Autodesk Inventor part; units mm, degrees
ref_plane "YZ Plane" through (0, 0, 0) normal (1, 0, 0) x (0, 1, 0)
ref_plane "XZ Plane" through (0, 0, 0) normal (0, 1, 0) x (-1, 0, 0)
ref_plane "XY Plane" through (0, 0, 0) normal (0, 0, 1) x (1, 0, 0)
ref_plane "Plano de trabajo1" through (0, 0, 0) normal (0, 0, 1) x (1, 0, 0)
sketch "Boceto1" plane through (0, 0, 0) normal (0, 0, 1) x (1, 0, 0)
  circle A0 centre (10.9923, 0) radius 10.9823
  circle A1 centre (10.9923, 0) radius 3.1378
  circle A2 centre (18.3423, 0) radius 1.2028
  circle A3 centre (10.9923, 7.35) radius 1.2028
  circle A4 centre (3.6423, 0) radius 1.2028
  circle A5 centre (10.9923, -7.35) radius 1.2028
  line L0 (0, 0) -> (0, 30)
  line L1 (21.9746, 0) -> (21.9746, -30)
  line L2 (0, 0) -> (0, -30)
  line L3 (0, -30) -> (21.9746, -30)
  circle A6 centre (10.9923, 0) radius 3.1378
  circle A7 centre (18.3423, 0) radius 1.2028
  circle A8 centre (10.9923, -7.35) radius 1.2028
  circle A9 centre (3.6423, 0) radius 1.2028
  circle A10 centre (10.9923, 7.35) radius 1.2028
  circle A11 centre (10.9923, 0) radius 10.9823
  line L4 (0, 0) -> (0, -30)
  line L5 (0, -30) -> (21.9746, -30)
  line L6 (21.9746, -30) -> (21.9746, 0)
  dimension "d0" = 30
  dimension "d1" = 30
extrude "Extrusión1" add sketch "Boceto1" along normal blind 3
sketch "Boceto2" plane through (10.9923, 0, 3) normal (0, 0, 1) x (1, 0, 0)
  circle A0 centre (0, 0) radius 10.9823
  line L0 (10.9823, 0) -> (10.9823, -30)
  line L1 (10.9823, -30) -> (-9.7118, -30)
  line L2 (-9.7118, -30) -> (-10.9923, 0)
  circle A1 centre (0, 0) radius 10.9823
  circle A2 centre (0, -7.35) radius 1.2028
  circle A3 centre (-7.35, 0) radius 1.2028
  circle A4 centre (0, 7.35) radius 1.2028
  circle A5 centre (7.35, 0) radius 1.2028
  circle A6 centre (0, 0) radius 3.1378
  point P0 (-10.9723, -0.4683)
  dimension "d4" = 30
extrude "Extrusión2" add sketch "Boceto2" against normal blind 3 contours L0 L1 L2 A0
sketch "Boceto3" plane through (0, 0, 0) normal (0, 0, -1) x (-1, 0, 0)
  point P0 (0, 0)
sketch "Boceto4" plane through (0, 0, 3) normal (0, 0, 1) x (1, 0, 0)
  point P0 (0, 0)
sketch "Boceto5" plane through (0, 0, 0) normal (0, 0, -1) x (-1, 0, 0)
  arc A0 (-0.02, -0.4683) -> (-21.9746, 0) centre (-10.9923, 0) ccw
  line L0 (-21.9746, 0) -> (-21.9746, -30)
  line L1 (-21.9746, -30) -> (-1.2805, -30)
  line L2 (-1.2805, -30) -> (-0.02, -0.4683)
  circle A1 centre (-10.9923, -7.35) radius 1.2028
  circle A2 centre (-3.6423, 0) radius 1.2028
  circle A3 centre (-10.9923, 7.35) radius 1.2028
  circle A4 centre (-18.3423, 0) radius 1.2028
  circle A5 centre (-10.9923, 0) radius 3.1378
  line L3 (-21.9746, -30) -> (0, -30)
  line L4 (0, -30) -> (0, 0)
  line L5 (0, 0) -> (-21.9746, 0)
  line L6 (-21.9746, 0) -> (-21.9746, -30)
  point P0 (-0.01, 0)
extrude "Extrusión3" add sketch "Boceto5" against normal blind 3 contours A0 L5 L4 L3 L2
sketch "Boceto6" plane through (0, 0, 0) normal (0, 0, -1) x (-1, 0, 0)
  point P0 (0, 0)
sketch "Boceto7" plane through (0, 0, 0) normal (0, 0, -1) x (-1, 0, 0)
  line L0 (-21.9746, -30) -> (0, -30)
  line L1 (-21.9746, -30) -> (-21.9746, 0)
  line L2 (0, -30) -> (-21.9746, -30)
  line L3 (-21.9746, -30) -> (-21.9746, -27)
  line L4 (-21.9746, -27) -> (0, -27)
  line L5 (0, -27) -> (0, -30)
  point P0 (0, 0)
  dimension "d9" = 3
extrude "Extrusión4" add sketch "Boceto7" along normal blind 40
sketch "Boceto8" plane through (0, -27, 0) normal (0, 1, 0) x (1, 0, 0)
  line L0 (0, -3) -> (0, 40)
  line L1 (21.9746, -3) -> (21.9746, 40)
  line L2 (0, 40) -> (21.9746, 40)
  line L3 (21.9746, 40) -> (21.9746, 38)
  line L4 (21.9746, 38) -> (0, 38)
  line L5 (0, 38) -> (0, 40)
  point P0 (0, 0)
  point P1 (21.9746, 40)
  point P2 (0, 38)
  dimension "d12" = 2
extrude "Extrusión5" add sketch "Boceto8" along normal blind 40
sketch "Boceto9" plane through (0, 0, -40) normal (0, 0, -1) x (-1, 0, 0)
  circle A0 centre (-11.0072, -0.015) radius 2.7
  circle A1 centre (-11.0099, -0.0117) radius 10.9823
  circle A2 centre (-18.3423, 0) radius 1.2028
  circle A3 centre (-10.9923, -7.35) radius 1.2028
  circle A4 centre (-10.9923, 7.35) radius 1.2028
  circle A5 centre (-3.6423, 0) radius 1.2028
  line L0 (-21.9746, -30) -> (-21.9746, 13)
  line L1 (-21.9746, -30) -> (0, -30)
  line L2 (0, -30) -> (0, 13)
  line L3 (-21.9746, 13) -> (0, 13)
  line L4 (-21.5706, 0) -> (-25.972, 0)
  line L5 (-25.972, 0) -> (-25.972, 18.1609)
  line L6 (-25.972, 18.1609) -> (4.5124, 18.1609)
  line L7 (4.5124, 18.1609) -> (4.5124, 1.2028)
  line L8 (4.5124, 1.2028) -> (4.5124, 0)
  line L9 (-3.6423, 0) -> (4.822, 0)
  point P0 (0, 0)
  point P1 (-21.9746, 0.6093)
  point P2 (-0.0276, 0)
  point P3 (0, 0)
extrude "Extrusión6" cut sketch "Boceto9" against normal blind 40 contours A0 | A1 L0 L3 L2 L9 | A2 | A3 | A4 | A5
sketch "Boceto10" plane through (0, -30, 3) normal (0, -1, 0) x (1, 0, 0)
  point P0 (0, -3)
sketch "Boceto11" plane through (0, -30, 3) normal (0, -1, 0) x (1, 0, 0)
  line L0 (0.0276, -43) -> (21.9746, -43)
  line L1 (0, -3) -> (0, 0)
  line L2 (21.9746, -43) -> (0, -43)
  line L3 (0, -43) -> (0, 0)
  line L4 (0, 0) -> (21.9746, 0)
  line L5 (21.9746, 0) -> (21.9746, -43)
  line L6 (0, -43) -> (-100, -43)
  line L7 (-100, -43) -> (-100, 0)
  line L8 (-100, 0) -> (0, 0)
  line L9 (0, 0) -> (0, -43)
  line L10 (-100, 0) -> (-100, -21.5)
  line L11 (-100, -21.5) -> (-100, -14.5)
  line L12 (-100, -14.5) -> (-100, -28.5)
  line L13 (-100, -28.5) -> (-50, -43)
  line L14 (-50, -43) -> (-50, 0)
  line L15 (-100, -14.5) -> (-50, 0)
  dimension "d17" = 100
  dimension "d18" = 21.5
  dimension "d19" = 7
  dimension "d20" = 14
extrude "Extrusión7" add sketch "Boceto11" along normal blind 10 contours L2 L3 L1 L4 L5 L0 | L6 L14 L8 L1 L3 | L13 L7 L15 L14
chamfer "Chaflán1" distance 2 angle 45 12 edges at (-14.0127, -40, -40) (-75, -40, -32.75) (-75, -30, -32.75) (-25, -30, -40) (-14.0127, -40, 3) (-75, -40, -4.25) (-100, -40, -18.5) (-75, -30, -4.25) (-25, -30, 3) (-100, -30, -18.5) (-100, -35, -25.5) (-100, -35, -11.5)
sketch "Boceto12" plane through (0, -40, 3) normal (0, -1, 0) x (1, 0, 0)
  line L0 (-49.7159, -2) -> (21.9746, -2)
  line L1 (-98, -16.0024) -> (-49.7159, -2)
  line L2 (-98, -26.9976) -> (-98, -16.0024)
  line L3 (-49.7159, -41) -> (-98, -26.9976)
  line L4 (21.9746, -41) -> (-49.7159, -41)
  line L5 (21.9746, -41) -> (21.9746, -2)
  line L6 (-48.5793, -33) -> (-88.2344, -21.5)
  line L7 (-88.2344, -21.5) -> (-48.5793, -10)
  line L8 (-48.5793, -10) -> (13.9746, -10)
  line L9 (13.9746, -10) -> (13.9746, -33)
  line L10 (13.9746, -33) -> (-48.5793, -33)
  point P0 (0, -3)
  dimension "d26" = 8
extrude "Extrusión8" cut sketch "Boceto12" against normal blind 4 contours L6 L7 L8 L9 L10
sketch "Boceto13" plane through (0, 0, -40) normal (0, 0, -1) x (-1, 0, 0)
  circle A0 centre (-11.0099, -0.0117) radius 5.6
  circle A1 centre (-11.0072, -0.015) radius 2.7
  point P0 (0, 0)
extrude "Extrusión9" cut sketch "Boceto13" against normal blind 5
sketch "Boceto14" plane through (0, 0, 0) normal (-1, 0, 0) x (0, 0, 1)
  line L0 (0, -27) -> (-38, -27)
  line L1 (-38, 0) -> (-40, 0)
  line L2 (-40, -32) -> (-40, 0)
  line L3 (-38, -30) -> (-40, -32)
  line L4 (1, -30) -> (-38, -30)
  line L5 (3, -32) -> (1, -30)
  line L6 (3, 0) -> (3, -32)
  line L7 (0, 0) -> (3, 0)
  line L8 (0, -27) -> (0, 0)
  line L9 (0, -27) -> (-38, -27)
  line L10 (-38, -27) -> (-38, 0)
  point P0 (0, 0)
extrude "Extrusión10" add sketch "Boceto14" along normal blind 30
sketch "Boceto15" plane through (0, 0, 3) normal (0, 0, 1) x (1, 0, 0)
  line L0 (21.9746, -38) -> (-50, -38)
  line L1 (21.9746, -38) -> (21.9746, 0)
  arc A0 (21.9746, 0) -> (0.01, 0) centre (10.9923, 0) ccw
  line L2 (0.01, 0) -> (-30, 0)
  line L3 (-30, -32) -> (-30, 0)
  line L4 (-50, -32) -> (-30, -32)
  line L5 (-50, -32) -> (-50, -38)
  circle A1 centre (10.9923, -7.35) radius 1.2028
  circle A2 centre (3.6423, 0) radius 1.2028
  circle A3 centre (10.9923, 7.35) radius 1.2028
  circle A4 centre (18.3423, 0) radius 1.2028
  circle A5 centre (10.9923, 0) radius 3.1378
  line L6 (21.9746, -27) -> (-30, -27)
  line L7 (0.01, 0) -> (-30, -27)
  point P0 (0, 0)
extrude "Extrusión11" cut sketch "Boceto15" against normal blind 100 contours L3 L2 L7
chamfer "Chaflán2" distance 2 angle 45 1 edges at (-30, -27, -19)
sketch "Boceto16" plane through (21.9746, -27, 0) normal (0, 1, 0) x (1, 0, 0)
  line L0 (-49.9746, 0) -> (-49.9746, 38)
  line L1 (0, 0) -> (-49.9746, 0)
  line L2 (0, 0) -> (0, 38)
  line L3 (0, 38) -> (-49.9746, 38)
  line L4 (0, 0) -> (-16, 0)
  line L5 (-16, 0) -> (-16, 6)
  line L6 (-16, 6) -> (0, 6)
  line L7 (0, 6) -> (0, 0)
  line L8 (0, 38) -> (-16, 38)
  line L9 (-16, 38) -> (-16, 32)
  line L10 (-16, 32) -> (0, 32)
  line L11 (0, 32) -> (0, 38)
  point P0 (-21.9746, 0)
  dimension "d38" = 16
  dimension "d39" = 6
  dimension "d40" = 16
  dimension "d41" = 6
extrude "Extrusión12" add sketch "Boceto16" along normal blind 6 contours L5 L6 L2 L1 | L3 L2 L10 L9
chamfer "Chaflán3" distance 6 angle 45 2 edges at (13.9746, -21, -6) (13.9746, -21, -32)
sketch "Boceto17" plane through (5.9746, -27, -38) normal (-1, 0, 0) x (0, 0, 1)
  line L0 (0, 6) -> (6, 0)
  line L1 (0, 0) -> (0, 6)
  line L2 (6, 0) -> (0, 0)
  line L3 (32, 0) -> (38, 6)
  line L4 (38, 0) -> (32, 0)
  line L5 (38, 6) -> (38, 0)
  point P0 (38, 27)
extrude "Extrusión13" add sketch "Boceto17" along normal blind 28
sketch "Boceto18" plane through (0, 0, -40) normal (0, 0, -1) x (-1, 0, 0)
  circle A0 centre (-10.9923, 0) radius 3.1378
  circle A1 centre (-11.0099, -0.0117) radius 5.6
  point P0 (0, 0)
extrude "Extrusión14" add sketch "Boceto18" against normal blind 2
properties part number "tibia"
Verification items for the finished model (mm, model axes). A direction names the side the tool comes from. Coordinates: 2 decimals unless noted, no trailing zeros. Order: outer loops, then holes, each group sorted by start corner. A loop starts at its lowest first (then second) coordinate and runs counter-clockwise, first axis right, second up. Notation, with made-up numbers: (54, 13) - (106, 13) arc R34 ccw to (106, 51) - close; hole circle Ø9 at (-29, 8.25). An arc over 180 degrees is marked (long way). Return JSON: item names as keys, results as strings.
(1) Section check A-A, the plane y = -34.5. Record the cut outline in (x, z), and give its area (3 significant figures).
Filled sheet:
{"outline": "(-100, -23.5) - (-98.08, -26.06) - (-50, -40) - (21.97, -40) - (21.97, 3) - (-50, 3) - (-98.08, -10.94) - (-100, -13.5) - close", "area": "4,520 mm^2"}
(2) Section check D-D, the plane z = -2. Record the cut outline in (x, y).
Filled sheet:
{"outline": "(-67.24, -38) - (-60.06, -40) - (21.97, -40) - (21.97, -23) - (-22.03, -23) - (-22.03, -27) - (-28, -27) - (-30, -29) - (-30, -30) - (-60.06, -30) - (-67.24, -32) - close"}
(3) Section check B-B, the plane x = -42.5. Record the cut outline in (y, z), and give its area (3 significant figures).
Filled sheet:
{"outline": "(-40, -38) - (-38, -40) - (-32, -40) - (-30, -38) - (-30, 1) - (-32, 3) - (-38, 3) - (-40, 1) - (-40, -7) - (-36, -7) - (-36, -30) - (-40, -30) - close", "area": "330 mm^2"}
(4) Mould release check, pull along Y, two halves, no side actions. Record for faces 1 (the cylindrical face through (12.103, 7.811, 1.479)), 2 (the flat face through (2, -9, -38)), 3 (the flat face through (0, -24, -35)): pulls with the +Y half, pulls with the -Y half, needs draft (parallel to the pull), parting line crosses it, or undercut.
Filled sheet:
{"face 1": "undercut", "face 2": "needs draft", "face 3": "pulls with the +Y half"}
(5) Thickness scan on line 1 along Z through (x, y) = (-26.5, -37.5); line 2 along Z through (x, y) = (7, 6); line 3 along Y through (x, z) = (-30.5, -37.5). Record the ranges inside material, lowest first.
Filled sheet:
{"line 1": "z = -40 to -30, -7 to 3", "line 2": "z = -40 to -38, 0 to 3", "line 3": "y = -40 to -30"}
(6) Access from +Z, -Z, +X, -X, +Y, -Y to the whole of each face (thin tool, end or side, straight path). Record for faces 4 (the flat face through (-17, -38, -30)), 5 (the flat face through (-57, -30, -18)), 6 (the flat face through (-74, -31, -5)), 7 (the flat face through (-22.025, -25, -36)), 8 (the cylindrical face through (8.094, -1.202, -39.014)).
Filled sheet:
{"face 4": "-Y", "face 5": "+Z, -Z, -X, +Y", "face 6": "+Z, -X, +Y", "face 7": "-X, +Y", "face 8": "+Z, -Z"}
(7) Go/stop test with flat-tipped pins: pin 1 (10 mm diameter, centred on x = 10.99, y = 0, fed in from -Z); pin 2 (3 mm diameter, centred on x = -69, z = -7.5, fed in from +Y); pin 3 (4 mm diameter, centred on y = -29, z = -22, fed in from -X). Record where each tip stops, or that it passes through.
Filled sheet:
{"pin 1": "stops at z = -40", "pin 2": "stops at y = -30", "pin 3": "stops at x = -99"}
(8) Section check C-C, the plane y = -15.5. Record the cut outline in (x, z), and give its area (3 significant figures).
Filled sheet:
{"outline": "(-17.22, -40) - (21.97, -40) - (21.97, -38) - (-17.22, -38) - close; (-17.22, 0) - (21.97, 0) - (21.97, 3) - (-17.22, 3) - close", "area": "196 mm^2"}
